Autodesk Fusion 360 part; units mm, degrees
sketch "Sketch1" plane through (0, 0, 0) normal (0, 0, 1) x (1, 0, 0) in component "Hackpad Case"
  line L0 (1, 47.0118) -> (84, 47.0118)
  line L1 (84, 47.0118) -> (84, -21.9882)
  line L2 (84, -21.9882) -> (1, -21.9882)
  line L3 (1, -21.9882) -> (1, 47.0118)
  line L4 (-7, 55.0118) -> (92, 55.0118)
  line L5 (92, 55.0118) -> (92, -29.9882)
  line L6 (92, -29.9882) -> (-7, -29.9882)
  line L7 (-7, -29.9882) -> (-7, 55.0118)
  circle A0 centre (-3, 51.0118) radius 2.35
  circle A1 centre (88, 51.0118) radius 2.35
  circle A2 centre (-3, -25.9882) radius 2.35
  circle A3 centre (88, -25.9882) radius 2.35
  circle A4 centre (4.9559, 43.136) radius 1.6
  line L8 (1, 47.0118) -> (9, 47.0118)
  line L9 (9, 47.0118) -> (9, 43.0118)
  line L10 (5, 39.0118) -> (1, 39.0118)
  line L11 (1, 39.0118) -> (1, 47.0118)
  circle A5 centre (79.9559, 43.136) radius 1.6
  line L12 (84, 47.0118) -> (76, 47.0118)
  line L13 (76, 47.0118) -> (76, 43.0118)
  line L14 (80, 39.0118) -> (84, 39.0118)
  line L15 (84, 39.0118) -> (84, 47.0118)
  circle A6 centre (4.9559, -17.864) radius 1.6
  line L16 (1, -21.9882) -> (9, -21.9882)
  line L17 (9, -21.9882) -> (9, -17.9882)
  line L18 (5, -13.9882) -> (1, -13.9882)
  line L19 (1, -13.9882) -> (1, -21.9882)
  line L20 (84, -21.9882) -> (76, -21.9882)
  line L21 (76, -21.9882) -> (76, -17.9882)
  line L22 (80, -13.9882) -> (84, -13.9882)
  line L23 (84, -13.9882) -> (84, -21.9882)
  circle A7 centre (79.9559, -17.864) radius 1.6
  arc A8 (5, 39.0118) -> (9, 43.0118) centre (5, 43.0118) ccw
  arc A9 (76, 43.0118) -> (80, 39.0118) centre (80, 43.0118) ccw
  arc A10 (80, -13.9882) -> (76, -17.9882) centre (80, -17.9882) ccw
  arc A11 (9, -17.9882) -> (5, -13.9882) centre (5, -17.9882) ccw
  point P0 (9, 39.0118)
  point P1 (76, 39.0118)
  point P2 (9, -13.9882)
  point P3 (76, -13.9882)
  dimension "d1" = 83
  dimension "d2" = 69
  dimension "d3" = 8
  dimension "d4" = 8
  dimension "d5" = 8
  dimension "d6" = 8
  dimension "d7" = 4.7
  dimension "d8" = 4
  dimension "d9" = 4
  dimension "d10" = 4.7
  dimension "d11" = 4
  dimension "d12" = 4
  dimension "d13" = 4.7
  dimension "d14" = 4
  dimension "d15" = 4
  dimension "d16" = 4.7
  dimension "d17" = 4
  dimension "d18" = 4
  dimension "d22" = 3.2
  dimension "d25" = 8
  dimension "d26" = 8
  dimension "d27" = 3.2
  dimension "d28" = 8
  dimension "d29" = 8
  dimension "d32" = 3.2
  dimension "d33" = 8
  dimension "d34" = 8
  dimension "d37" = 8
  dimension "d38" = 8
  dimension "d39" = 3.2
  dimension "d62" = 61
  dimension "d63" = 75
  dimension "d64" = 75
  dimension "d65" = 61
  dimension "d66" = 4
  dimension "d67" = 4
  dimension "d68" = 4
  dimension "d69" = 4
extrude "Extrude1" add sketch "Sketch1" along normal blind 3 contours L0 L3 L8 L9 L10 L11 A8 | L0 L1 L2 L3 L9 L10 L13 L14 L17 L18 L21 L22 A8 A9 A10 A11 | L0 L1 L12 L13 L14 L15 A9 | L2 L3 L16 L17 L18 L19 A11 | L1 L2 L20 L21 L22 L23 A10 | L4 L5 L6 L7 | A0 | A1 | A2 | A3
extrude "Extrude2" add sketch "Sketch1" along normal blind 18.5 contours L4 L5 L6 L7
extrude "Extrude3" add sketch "Sketch1" along normal blind 12.31 contours L0 L3 L8 L9 L10 L11 A8 | L0 L1 L12 L13 L14 L15 A9 | L2 L3 L16 L17 L18 L19 A11 | L1 L2 L20 L21 L22 L23 A10
sketch "Sketch3" plane through (0, 0, 18.5) normal (0, 0, 1) x (-1, 0, 0)
  line L0 (-84, -47.0118) -> (-84, 21.9882)
  line L1 (-84, 21.9882) -> (-1, 21.9882)
  line L2 (-1, 21.9882) -> (-1, -47.0118)
  line L3 (-1, -47.0118) -> (-84, -47.0118)
  circle A0 centre (3, 25.9882) radius 2.35
  circle A1 centre (-88, 25.9882) radius 2.35
  circle A2 centre (-88, -51.0118) radius 2.35
  circle A3 centre (3, -51.0118) radius 2.35
  line L4 (7, 29.9882) -> (-92, 29.9882)
  line L5 (-92, 29.9882) -> (-92, -55.0118)
  line L6 (-92, -55.0118) -> (7, -55.0118)
  line L7 (7, -55.0118) -> (7, 29.9882)
  line L8 (7, -38.636) -> (-1, -38.636)
  line L9 (-1, -38.636) -> (-1, -22.636)
  line L10 (-1, -22.636) -> (7, -22.636)
  line L11 (7, -22.636) -> (7, -38.636)
  circle A4 centre (-4.9559, -43.136) radius 1.6
  circle A5 centre (-4.9559, 17.864) radius 1.6
  dimension "d78" = 4.5
  dimension "d79" = 40.5
extrude "Extrude4" cut sketch "Sketch3" against normal blind 8 contours L2 L7 L8 L9 L10 L11
fillet "Fillet2" radius 4 4 edges at (-7, -29.9882, 9.25) (92, -29.9882, 9.25) (92, 55.0118, 9.25) (-7, 55.0118, 9.25)
fillet "Fillet3" radius 2 2 edges at (-3, 22.636, 10.5) (-3, 38.636, 10.5)
fillet "Fillet4" radius 1 10 edges at (-7, 22.636, 15.5) (-7, 23.2217, 11.0858) (-7, 30.636, 10.5) (-7, 38.0502, 11.0858) (-7, 38.636, 15.5) (1, 38.636, 15.5) (1, 38.0502, 11.0858) (1, 30.636, 10.5) (1, 23.2217, 11.0858) (1, 22.636, 15.5)
component "Hackpad Case" placed x (1, 0, 0) y (0, 1, 0) z (0, 0, 1) at (0, 0, 0)
For this review, take the finished solid that the model builds, in its own axes (mm). A direction names the side the tool comes from. Give positions to 0.01 mm unless a question says otherwise; leave off trailing zeros. Order: outer loops, then holes, each group sorted by start corner. A loop starts at its lowest first (then second) coordinate and runs counter-clockwise, first axis right, second up.
1) The part is to be moulded in two halves that separate along Y. For faces 1 (the face through (82, 39.012, 8)), 2 (the face through (90.859, -28.785, 9.12)), 3 (the face through (-3, 31, 10.5)), say which applies: released by +Y, released by -Y, zero draft, split by the parting line, or undercut.
2) Take a section at A-A (y = 10.5). Give the boundary of the cut face in (x, z), then the cut area to 3 significant figures.
3) Wall thickness on line 1 (Y direction, x = 88, z = 14.25); line 2 (X direction, y = -26, z = 4.75); line 3 (X direction, y = 29, z = 5): over which ranges is each line inside the solid? List them lowest first.
4) Take a section at B-B (x = 27.5). Give the boundary of the cut face in (y, z).
5) Take a section at C-C (z = 4.5). State how many separate pieces and enclosed holes the cut face has, then the cut area to 3 significant figures.
6) For faces 4 (the face through (77.14, -15.19, 7.59)), 5 (the face through (-3, 22.636, 16)), 6 (the face through (78.686, -16.89, 6.069)), list the 3-axis set-ups (+Z, -Z, +X, -X, +Y, -Y) from which the entire face can be reached by the end or side of a thin tool; tool diameter is ignored.
7) Insertion check: pin 1 (1 mm diameter, centred on x = 7.5, y = 6, fed in from -Z); pin 2 (4 mm diameter, centred on x = 79.5, y = 44.5, fed in from +Z). Each pin has a flat end and moves straight along its axis. Give the tip position at first contact, or say it passes through.
Derived:
1. face 1: undercut
1. face 2: released by -Y
1. face 3: undercut
2. outline: (-7, 0) - (92, 0) - (92, 18.5) - (84, 18.5) - (84, 3) - (1, 3) - (1, 18.5) - (-7, 18.5) - close
2. area: 545 mm2
3. line 1: y = -29.99 to -28.34, -23.64 to 48.66, 53.36 to 55.01
3. line 2: x = -7 to -5.35, -0.65 to 85.65, 90.35 to 92
3. line 3: x = -7 to 1, 84 to 92
4. outline: (-29.99, 0) - (55.01, 0) - (55.01, 18.5) - (47.01, 18.5) - (47.01, 3) - (-21.99, 3) - (-21.99, 18.5) - (-29.99, 18.5) - close
5. separate pieces: 1
5. enclosed holes: 9
5. area: 2,810 mm2
6. face 4: +Z
6. face 5: +Z, -X
6. face 6: +Z, -Z
7. pin 1: stops at z = 0
7. pin 2: stops at z = 12.31
